from build123d import *

# Parameters (mm, degrees)
F0_W     = 30.48
F0_H     = 95.25
F0_R     = 6.35
F0_W_2   = 5.08
F0_H_2   = 5.08
F1_DEPTH = 25.4
F2_R     = 6.35
F3_DEPTH = 95.251


with BuildPart() as f1:
    # F0 (on Front) → F1 (new body)
    with BuildSketch(Plane.XZ):
        with Locations((-275.705503, 4.959305)):
            Rectangle(F0_W, F0_H)
        with Locations((-275.705503, -17.265695)):
            Circle(F0_R, mode=Mode.SUBTRACT)
        with Locations((-275.705503, 27.184305)):
            Rectangle(F0_W_2, F0_H_2, mode=Mode.SUBTRACT)
    extrude(amount=F1_DEPTH)

    # F2 (on face) → F3 (cut, through all)
    with BuildSketch(Plane(origin=(0, 0, -42.665695), x_dir=(1, 0, 0), z_dir=(0, 0, -1))):
        with Locations((-275.705503, 13.97)):
            Circle(F2_R)
    extrude(amount=-F3_DEPTH, mode=Mode.SUBTRACT)


solid = f1.part
Can you work these out from the model? Positions are in its coordinate system, mm. A direction names the side the tool comes from. Give positions to 0.01 mm unless a question says otherwise; leave off trailing zeros. Write each loop counter-clockwise with the first axis right and the second up, starting at its lowest first coordinate (ties: lowest second). Pieces come first, ordered by that corner, then holes. Notation, with made-up numbers: M 2,56 L 16,56 A26 ccw 16,74 Z; hole C -8,-4.75 d5. An arc over 180 degrees is marked long. Answer in a Markdown table with one row per item. Add a question column.
Item 1: We'd pull the mould along Z, two halves only. Please class faces 1 (the flat face through (-276, -25.4, 6)), 2 (the flat face through (-276, -4, 24.644)), 3 (the flat face through (-276, -7, -42.666)): released by +Z, released by -Z, zero draft, split by the parting line, or undercut.
Item 2: For pin 1 Ø7.5 at (x, z) = (-275.71, -17.27) entering from +Y, with a flat end and sliding along its axis, tell me the tip position at first contact or that it passes through.
Item 3: Imagine slicing it at C-C, the plane z = 36. Write out the boundary of the cut face in (x, y), plus the area to 3 significant figures.
Item 4: Imagine slicing it at D-D, the plane x = -281. Write out the boundary of the cut face in (y, z).
Item 5: Imagine slicing it at B-B, the plane y = -18.5. Write out the boundary of the cut face in (x, z).
Item 6: On a 3-axis mill with a long thin cutter (end or side, diameter ignored), from which of +Z, -Z, +X, -X, +Y, -Y can I reach the whole of each face in a straight line? I mean faces 4 (the flat face through (-278.246, -4, 27)), 5 (the flat face through (-276, -7, 52.584)). Say none if no direction works.
Item 7: Imagine slicing it at A-A, the plane z = -19. Write out the boundary of the cut face in (x, y), plus the area to 3 significant figures.
Item 8: Please list where these lines run through material, in increasing order: L1, parallel to Z at x = -275.5, y = -5; L2, parallel to Z at x = -277.5, y = -5.75; L3, parallel to X at y = -13.97, z = -24.5.
Evaluation:
| question | item | result |
|---|---|---|
| 1 | face 1 | zero draft |
| 1 | face 2 | undercut |
| 1 | face 3 | released by -Z |
| 2 | pin 1 | passes through |
| 3 | outline | M -290.95,-25.4 L -260.47,-25.4 L -260.47,0 L -290.95,0 Z; hole C -275.71,-13.97 d12.7 |
| 3 | area | 648 mm² |
| 4 | outline | M -25.4,-42.67 L -17.48,-42.67 L -17.48,-20.77 L -25.4,-20.77 Z; M -25.4,-13.76 L -17.48,-13.76 L -17.48,52.58 L -25.4,52.58 Z; M -10.46,-42.67 L 0,-42.67 L 0,-20.77 L -10.46,-20.77 Z; M -10.46,-13.76 L 0,-13.76 L 0,52.58 L -10.46,52.58 Z |
| 5 | outline | M -290.95,-42.67 L -280.16,-42.67 L -280.16,-21.8 A6.35 cw -280.16,-12.74 L -280.16,52.58 L -290.95,52.58 Z; M -271.26,-42.67 L -260.47,-42.67 L -260.47,52.58 L -271.26,52.58 L -271.26,-12.74 A6.35 cw -271.26,-21.8 Z |
| 6 | face 4 | +Y, -Y |
| 6 | face 5 | +Z, +X, -X, +Y, -Y |
| 7 | outline | M -290.95,-25.4 L -281.81,-25.4 L -281.81,-15.7 A6.35 cw -281.81,-12.24 L -281.81,0 L -290.95,0 Z; M -269.6,-25.4 L -260.47,-25.4 L -260.47,0 L -269.6,0 L -269.6,-12.24 A6.35 cw -269.6,-15.7 Z |
| 7 | area | 463 mm² |
| 8 | L1 | z = -42.67 to -23.61, -10.92 to 24.64, 29.72 to 52.58 |
| 8 | L2 | z = -42.67 to -23.36, -11.17 to 24.64, 29.72 to 52.58 |
| 8 | L3 | x = -290.95 to -282.06, -269.36 to -260.47 |
